```python
from build123d import *

# Parameters (mm, degrees)
BASE_FLANGE1_DEPTH                                = 2
SKETCH7_R                                         = 2
CUT_EXTRUDE1_DEPTH                                = 2
CSK_FOR_4_FLAT_HEAD_MACHINE_SCREW_100_D           = 3.2639
CSK_FOR_4_FLAT_HEAD_MACHINE_SCREW_100_DEPTH       = 2
CSK_FOR_4_FLAT_HEAD_MACHINE_SCREW_100_CSINK_D     = 5.715
CSK_FOR_4_FLAT_HEAD_MACHINE_SCREW_100_CSINK_ANGLE = 100
CSK_FOR_4_FLAT_HEAD_MACHINE_SCREW_100_TIP         = 0.980574487


# Sheet-metal steps are written as plain solids
with BuildPart() as part:
    # Sketch2 → Base-Flange1 (new body)
    with BuildSketch(Plane(origin=(0, 0, 0), x_dir=(1, 0, 0), z_dir=(0, 1, 0))):
        with BuildLine():
            Line((-26.055569119, -21.875), (-26.055569119, -46.875))
            Line((-26.055569119, -46.875), (-16.055569119, -46.875))
            Line((-16.055569119, -46.875), (-16.055569119, -21.875))
            Line((-16.055569119, -21.875), (26.055569119, -21.875))
            Line((26.055569119, -21.875), (26.055569119, 8.188046441))
            ThreePointArc((26.055569119, 8.188046441), (21.514872246, 4.669726518), (15.870079226, 5.73406431))
            ThreePointArc((15.870079226, 5.73406431), (10.616247764, 4.133629141), (7, 0))
            ThreePointArc((7, 0), (0, -7), (-7, 0))
            ThreePointArc((-7, 0), (-10.616247764, 4.133629141), (-15.870079226, 5.73406431))
            ThreePointArc((-15.870079226, 5.73406431), (-21.514872246, 4.669726518), (-26.055569119, 8.188046441))
            Line((-26.055569119, 8.188046441), (-26.055569119, -21.875))
        make_face()
    extrude(amount=-BASE_FLANGE1_DEPTH)

    # Sketch7 → Cut-Extrude1 (cut)
    with BuildSketch(Plane(origin=(0, 0, 0), x_dir=(1, 0, 0), z_dir=(0, 1, 0))):
        with Locations(Location((-21.055569119, -40.375, 0), (0, 0, 270))):
            Circle(SKETCH7_R)
        with Locations(Location((-21.055569119, -30.875, 0), (0, 0, 270))):
            Circle(SKETCH7_R)
    extrude(amount=-CUT_EXTRUDE1_DEPTH, mode=Mode.SUBTRACT)

    # CSK for #4 Flat Head Machine Screw (100)1
    with Locations(Plane(origin=(0, 0, 0), x_dir=(1, 0, 0), z_dir=(0, 1, 0))):
        with Locations((-7.875283017, -16.875), (7.875283017, -16.875)):
            CounterSinkHole(CSK_FOR_4_FLAT_HEAD_MACHINE_SCREW_100_D / 2, CSK_FOR_4_FLAT_HEAD_MACHINE_SCREW_100_CSINK_D / 2, depth=CSK_FOR_4_FLAT_HEAD_MACHINE_SCREW_100_DEPTH, counter_sink_angle=CSK_FOR_4_FLAT_HEAD_MACHINE_SCREW_100_CSINK_ANGLE)
            with Locations((0, 0, -(CSK_FOR_4_FLAT_HEAD_MACHINE_SCREW_100_DEPTH + CSK_FOR_4_FLAT_HEAD_MACHINE_SCREW_100_TIP / 2))):  # 118° drill point
                Cone(0, CSK_FOR_4_FLAT_HEAD_MACHINE_SCREW_100_D / 2, CSK_FOR_4_FLAT_HEAD_MACHINE_SCREW_100_TIP, mode=Mode.SUBTRACT)


solid = part.part
```
Part model, mm, in its own coordinate system. A direction names the side the tool comes from. Round coordinates to 2 decimals unless told otherwise and drop trailing zeros. Loops run counter-clockwise (first coordinate to the right, second up) from the corner with the lowest first, then second, coordinate; pieces in that order, holes last.
Item 1: Cut at A-A, the plane z = -2. Give the cut face in (x, y), then the cut area to 3 significant figures.
Item 2: Mould opens along Z. For faces 4 (the face through (-20.45, -0.99, 32.78)), 5 (the face through (21.6, -0.99, -4.69)), 6 (the face through (-6.245, -1.521, 16.803)), 7 (the face through (5, -1, 21.875)) say: +Z half, -Z half, draft (parallel to the pull), parting line (faces both ways), or undercut.
Item 3: Drill centre lines: line 1 (X direction, y = -0.15, z = 15); line 2 (X direction, y = -1.4, z = 23.5); line 3 (X direction, y = -1.7, z = 1). Where is each one in solid material? Low to high.
Item 4: 3-axis set-ups, long thin cutter, end or side, ignore diameter. For faces 1 (the face through (-10.55, -0.99, -4.09)), 2 (the face through (-19.073, -0.986, 40.115)), 3 (the face through (-16.056, -1, 35)): which of +Z, -Z, +X, -X, +Y, -Y reach the whole face in a straight line?
Item 5: Drop flat-ended pins along their axis: P1, Ø1, axis at y = -1.5, z = 33.5, coming from the +X side; P2, Ø1, axis at x = 9.5, y = -2, coming from the +Z side (3 decimals). Give the stop position or say it passes through.
Item 6: Cut at D-D, the plane x = -13. Give the cut face in (y, z) (3 decimals).
Item 7: Cut at C-C, the plane x = 0. Give the cut face in (y, z) (3 decimals).
Item 8: Cut at B-B, the plane y = -0.6. Give the cut face in (x, z) (3 decimals).
A:
1. outline: (-26.06, -2) - (-8.25, -2) - (-8.25, 0) - (-26.06, 0) - close; (8.25, -2) - (26.06, -2) - (26.06, 0) - (8.25, 0) - close
1. area: 71.2 mm2
2. face 4: undercut
2. face 5: -Z half
2. face 6: undercut
2. face 7: +Z half
3. line 1: x = -26.06 to -9.79, -5.96 to 5.96, 9.79 to 26.06
3. line 2: x = -26.06 to -16.06
3. line 3: x = -26.06 to -6.93, 6.93 to 26.06
4. face 1: -Z, +Y, -Y
4. face 2: +Y, -Y
4. face 3: +Z, +X, +Y, -Y
5. P1: stops at x = -16.06
5. P2: stops at z = 21.875
6. outline: (-2, -5.261) - (0, -5.261) - (0, 21.875) - (-2, 21.875) - close
7. outline: (-2, 7) - (0, 7) - (0, 21.875) - (-2, 21.875) - close
8. outline: (-26.056, -8.188) arc R7 cw to (-15.87, -5.734) arc R10 ccw to (-7, 0) arc R7 cw to (7, 0) arc R10 ccw to (15.87, -5.734) arc R7 cw to (26.056, -8.188) - (26.056, 21.875) - (-16.056, 21.875) - (-16.056, 46.875) - (-26.056, 46.875) - close; hole circle Ø4 at (-21.056, 30.875); hole circle Ø4 at (-21.056, 40.375); hole circle Ø4.285 at (-7.875, 16.875); hole circle Ø4.285 at (7.875, 16.875)
